For this review, take the finished solid that the model builds, in its own axes (mm). Face numbers are marked on the shaded views. A direction names the side the tool comes from. Give positions to 0.01 mm unless a question says otherwise; leave off trailing zeros. Loops run counter-clockwise (first coordinate to the right, second up) from the corner with the lowest first, then second, coordinate; pieces in that order, holes last. Notation, with made-up numbers: M 54,77.5 L 82,77.5 A11 ccw 82,92.5 Z; hole C 56.5,22 d9. An arc over 180 degrees is marked long. Use CSV: the item, a comma, the result in double quotes. Start each with the question number.
1. Insertion check: P1, Ø1.5, axis at x = -2, z = 5, coming from the -Y side; P2, Ø1.5, axis at y = 12, z = 2, coming from the +X side. Each pin has a flat end and moves straight along its axis. Give the tip position at first contact, or say it passes through.
2. Take a section at C-C, the plane z = -2.75. Write out the cut boundary in (x, y), and give its area (3 significant figures).
3. Tool access review of the marked faces 4, 5 and 6: name each direction out of +Z, -Z, +X, -X, +Y, -Y from which nothing blocks a thin tool from reaching the whole face with its end or side.
4. The part is to be moulded in two halves that separate along Z. For the marked faces 1, 2 and 3, say which applies: pulls with the +Z half, pulls with the -Z half, needs draft (parallel to the pull), parting line crosses it, or undercut.
5. Take a section at A-A, the plane x = 0. Write out the cut boundary in (y, z).
6. To check wall thickness, follow line 1 (Z direction, x = 6, y = -13); line 2 (Y direction, x = 0, z = -1.5); line 3 (Z direction, x = 9.75, y = 3.75). State the ranges of each line that lie inside material, in increasing order. Write a range as [from, to].
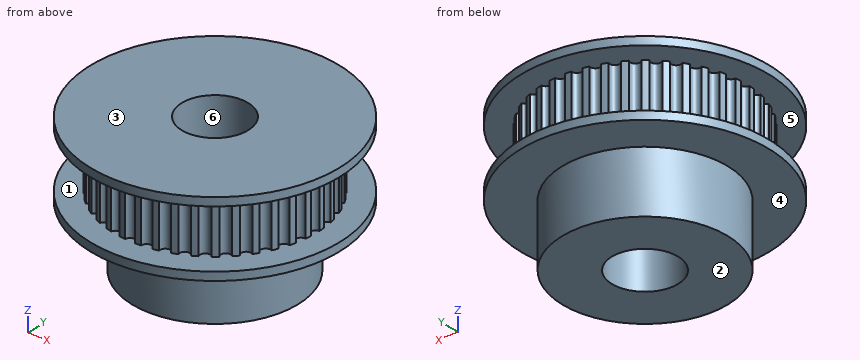
from build123d import *

# Parameters (mm, degrees)
SKETCH_1_R               = 15
EXTRUDE_1_DEPTH          = 0.5
SKETCH_2_R               = 12.23
EXTRUDE_2_DEPTH          = 7
SKETCH_8_R               = 10
EXTRUDE_4_DEPTH          = 8
CUT_EXTRUDE_3_DEPTH      = 7
SKETCH_3_R               = 15
EXTRUDE_3_DEPTH          = 1
SKETCH_6_R               = 4
CUT_EXTRUDE_2_DEPTH      = 8.5
CUT_EXTRUDE_2_DEPTH_BACK = 10
PATTERN_CIRCULAR_2_COUNT = 40


with BuildPart() as part:
    # 草圖1 → 填料-伸長1 (new body, symmetric)
    with BuildSketch(Plane.XY):
        Circle(SKETCH_1_R)
    extrude(amount=EXTRUDE_1_DEPTH, both=True)

    # 草圖2 → 填料-伸長2 (add)
    with BuildSketch(Plane.XY.offset(0.5)):
        Circle(SKETCH_2_R)
    extrude(amount=EXTRUDE_2_DEPTH)

    # 草圖8 → 填料-伸長4 (add)
    with BuildSketch(Plane(origin=(0, 0, 0), x_dir=(-1, 0, 0), z_dir=(0, 0, -1))):
        Circle(SKETCH_8_R)
    extrude(amount=EXTRUDE_4_DEPTH)

    # 草圖7 → 除料-伸長3 (cut)
    with BuildSketch(Plane.XY.offset(7.5)):
        with BuildLine():
            ThreePointArc((-0.599819459, 12.215282093), (0, 11.63), (0.599819459, 12.215282093))
            ThreePointArc((0.599819459, 12.215282093), (0, 12.23), (-0.599819459, 12.215282093))
        make_face()
    cut_extrude_3 = extrude(amount=-CUT_EXTRUDE_3_DEPTH, mode=Mode.SUBTRACT)

    # 草圖3 → 填料-伸長3 (add)
    with BuildSketch(Plane.XY.offset(7.5)):
        Circle(SKETCH_3_R)
    extrude(amount=EXTRUDE_3_DEPTH)

    # 草圖6 → 除料-伸長2 (cut, two sides)
    with BuildSketch(Plane(origin=(0, 0, -0.5), x_dir=(-1, 0, 0), z_dir=(0, 0, -1))) as cut_extrude_2_sk:
        Circle(SKETCH_6_R)
    extrude(amount=CUT_EXTRUDE_2_DEPTH, mode=Mode.SUBTRACT)
    extrude(cut_extrude_2_sk.sketch, amount=-CUT_EXTRUDE_2_DEPTH_BACK, mode=Mode.SUBTRACT)

    # 環狀複製排列2: 除料-伸長3 ×40 about axis
    pattern_circular_2_axis = Axis((0, 0, 0), (0, 0, 1))
    for i in range(1, PATTERN_CIRCULAR_2_COUNT):
        add(cut_extrude_3.rotate(pattern_circular_2_axis, i * 360 / PATTERN_CIRCULAR_2_COUNT), mode=Mode.SUBTRACT)


solid = part.part
Result set:
1,P1,"y = -12.17"
1,P2,"x = 4.8"
2,outline,"C 0,0 d20; hole C 0,0 d8"
2,area,"264 mm2"
3,face 4,"-Z"
3,face 5,"none"
3,face 6,"+Z, -Z"
4,face 1,"undercut"
4,face 2,"pulls with the -Z half"
4,face 3,"pulls with the +Z half"
5,outline,"M -15,-0.5 L -10,-0.5 L -10,-8 L -4,-8 L -4,8.5 L -15,8.5 L -15,7.5 L -11.63,7.5 L -11.63,0.5 L -15,0.5 Z; M 4,-8 L 10,-8 L 10,-0.5 L 15,-0.5 L 15,0.5 L 11.63,0.5 L 11.63,7.5 L 15,7.5 L 15,8.5 L 4,8.5 Z"
6,line 1,"[-0.5, 0.5], [7.5, 8.5]"
6,line 2,"[-10, -4], [4, 10]"
6,line 3,"[-0.5, 8.5]"
